Build history of the part. All positions in model axes, mm. Face numbers are marked on the shaded views. A direction names the side the tool comes from. Coordinates: 2 decimals unless noted, no trailing zeros. Loops run counter-clockwise (first coordinate to the right, second up) from the corner with the lowest first, then second, coordinate; pieces in that order, holes last.
Item 1: Cut at C-C (x = -15). List the corners of the cut face in (y, z).
Item 2: Drill centre lines: line 1 along X through (y, z) = (45, 39); line 2 along Y through (x, z) = (-16.5, 40); line 3 along Z through (x, y) = (-122, 45.5). Where is each one in solid material? Low to high.
Item 3: Mould opens along Y. For the marked faces 1, 2, 3 and 4 say: released by +Y, released by -Y, zero draft, split by the parting line, or undercut.
Item 4: Cut at B-B (y = 39.5). List the corners of the cut face in (x, z).
Item 5: Cut at A-A (z = 16.5). List the corners of the cut face in (x, y), and give its area (3 significant figures).
Item 6: Flat gauge pin, fed straight in: pin 1 (22 mm diameter, centred on x = -90.5, y = 32, fed in from +Z). Where does the tip first touch, or does it go through?
Item 7: Cut at D-D (z = 8.5). List the corners of the cut face in (x, y), and give its area (3 significant figures).
Item 8: 3-axis set-ups, long thin cutter, end or side, ignore diameter. For the marked faces 5 and 6: which of +Z, -Z, +X, -X, +Y, -Y reach the whole face in a straight line?
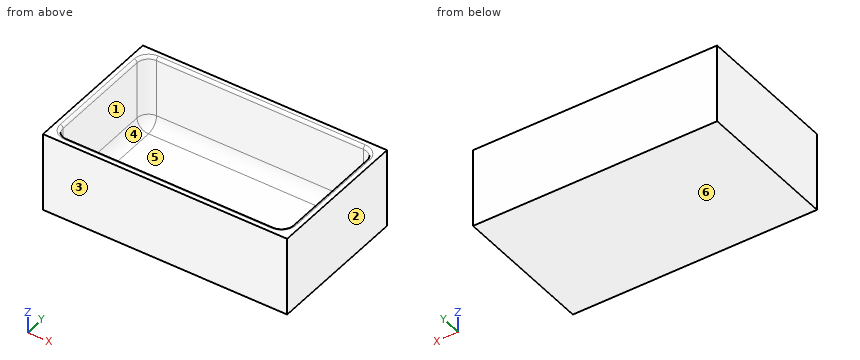
from build123d import *

# Parameters (mm, degrees)
IZIM1_W                     = 90
IZIM1_H                     = 160
Y_KSEKLIK_EKSTR_ZYON1_DEPTH = 5
IZIM1_3_W                   = 100
IZIM1_3_H                   = 170
IZIM1_3_W_2                 = 90
IZIM1_3_H_2                 = 160
Y_KSEKLIK_EKSTR_ZYON2_DEPTH = 55
RADYUS1_R                   = 8
RADYUS2_R                   = 2


with BuildPart() as part:
    # Çizim1 → Yükseklik-Ekstrüzyon1 (new body)
    with BuildSketch(Plane(origin=(0, 0, 0), x_dir=(0, 1, 0), z_dir=(0, 0, 1))):
        with Locations((50, 85)):
            Rectangle(IZIM1_W, IZIM1_H)
    extrude(amount=Y_KSEKLIK_EKSTR_ZYON1_DEPTH)

    # Çizim1<3> → Yükseklik-Ekstrüzyon2 (add)
    with BuildSketch(Plane(origin=(0, 0, 0), x_dir=(0, 1, 0), z_dir=(0, 0, 1))):
        with Locations((50, 85)):
            Rectangle(IZIM1_3_W, IZIM1_3_H)
        with Locations((50, 85)):
            Rectangle(IZIM1_3_W_2, IZIM1_3_H_2, mode=Mode.SUBTRACT)
    extrude(amount=Y_KSEKLIK_EKSTR_ZYON2_DEPTH)

    # Radyus1
    radyus1_edges = [part.edges().sort_by_distance(p)[0] for p in [
        (-165, 50, 5),
        (-5, 95, 30),
        (-165, 95, 30),
        (-165, 5, 30),
        (-5, 5, 30),
        (-85, 5, 5),
        (-5, 50, 5),
        (-85, 95, 5),
    ]]
    fillet(radyus1_edges, radius=RADYUS1_R)

    # Radyus2
    radyus2_edges = [part.edges().sort_by_distance(p)[0] for p in [
        (-5, 50, 55),
        (-85, 95, 55),
        (-85, 5, 55),
        (-165, 50, 55),
        (-7.343145751, 92.656854249, 55),
        (-7.343145751, 7.343145751, 55),
        (-162.656854249, 92.656854249, 55),
        (-162.656854249, 7.343145751, 55),
    ]]
    fillet(radyus2_edges, radius=RADYUS2_R)


solid = part.part
Filled sheet:
1. outline: (0, 0) - (100, 0) - (100, 55) - (97, 55) arc R2 ccw to (95, 53) - (95, 13) arc R8 cw to (87, 5) - (13, 5) arc R8 cw to (5, 13) - (5, 53) arc R2 ccw to (3, 55) - (0, 55) - close
2. line 1: x = -170 to -165, -5 to 0
2. line 2: y = 0 to 5, 95 to 100
2. line 3: z = 0 to 5
3. face 1: undercut
3. face 2: zero draft
3. face 3: released by -Y
3. face 4: undercut
4. outline: (-170, 0) - (0, 0) - (0, 55) - (-3, 55) arc R2 ccw to (-5, 53) - (-5, 13) arc R8 cw to (-13, 5) - (-157, 5) arc R8 cw to (-165, 13) - (-165, 53) arc R2 ccw to (-167, 55) - (-170, 55) - close
5. outline: (-170, 0) - (0, 0) - (0, 100) - (-170, 100) - close; hole (-165, 13) arc R8 ccw to (-157, 5) - (-13, 5) arc R8 ccw to (-5, 13) - (-5, 87) arc R8 ccw to (-13, 95) - (-157, 95) arc R8 ccw to (-165, 87) - close
5. area: 2,650 mm2
6. pin 1: stops at z = 5
7. outline: (-170, 0) - (0, 0) - (0, 100) - (-170, 100) - close; hole (-163.61, 13) arc R6.61 ccw to (-157, 6.39) - (-13, 6.39) arc R6.61 ccw to (-6.39, 13) - (-6.39, 87) arc R6.61 ccw to (-13, 93.61) - (-157, 93.61) arc R6.61 ccw to (-163.61, 87) - close
7. area: 3,320 mm2
8. face 5: +Z
8. face 6: -Z, +X, -X, +Y, -Y
